```python
from build123d import *

# Parameters (mm, degrees)
BOSS_EXTRUDE1_DEPTH     = 7
BOSS_EXTRUDE2_OUTLINE_R = 32.5
BOSS_EXTRUDE2_DEPTH     = 5
CUT_EXTRUDE1_START      = -10
CUT_EXTRUDE1_DEPTH      = 10
CIRPATTERN1_COUNT       = 12


# Read off the part's stored shape, not the designer's step: Boss-Extrude2, CBORE for M3 SHCS1
with BuildPart() as part:
    # Sketch1 → Boss-Extrude1 (new body)
    with BuildSketch(Plane.XY):
        with BuildLine():
            Line((0, 0), (-0.403978912, 15.69480172))
            ThreePointArc((-0.403978912, 15.69480172), (-9.850874058, 16.938509061), (-18.653978912, 20.584874482))
            ThreePointArc((-18.653978912, 20.584874482), (-20.11149054, 20.82324131), (-21.567676923, 20.576907974))
            ThreePointArc((-21.567676923, 20.576907974), (-24.205855638, 20.575365577), (-26.541253498, 21.802519254))
            ThreePointArc((-26.541253498, 21.802519254), (-28.493972378, 23.657335535), (-30.31737883, 25.639416102))
            ThreePointArc((-30.31737883, 25.639416102), (-31.544532507, 27.974813962), (-31.54299011, 30.612992677))
            ThreePointArc((-31.54299011, 30.612992677), (-31.455305934, 32.324569937), (-32.01390615, 33.94480172))
            Line((-32.01390615, 33.94480172), (-51.738215412, 33.94480172))
            ThreePointArc((-51.738215412, 33.94480172), (-38.72021408, 13.062776736), (-17.866169147, 0))
            Line((-17.866169147, 0), (0, 0))
        make_face()
        with BuildLine():
            ThreePointArc((17.846021088, 20.584874482), (9.042916235, 16.938509061), (-0.403978912, 15.69480172))
            Line((-0.403978912, 15.69480172), (0, 0))
            Line((0, 0), (17.866169147, 0))
            ThreePointArc((17.866169147, 0), (38.72021408, 13.062776736), (51.738215412, 33.94480172))
            Line((51.738215412, 33.94480172), (31.205948327, 33.94480172))
            ThreePointArc((31.205948327, 33.94480172), (30.756396425, 32.859487423), (30.603062644, 31.69480172))
            ThreePointArc((30.603062644, 31.69480172), (30.636176894, 31.149887325), (30.735032287, 30.612992677))
            ThreePointArc((30.735032287, 30.612992677), (30.855855546, 29.956788108), (30.896328518, 29.290781625))
            ThreePointArc((30.896328518, 29.290781625), (30.537924024, 27.337836245), (29.509421007, 25.639416102))
            ThreePointArc((29.509421007, 25.639416102), (27.880292336, 23.910530473), (26.151406706, 22.281401802))
            ThreePointArc((26.151406706, 22.281401802), (23.816008846, 21.054248125), (21.177830131, 21.055790522))
            ThreePointArc((21.177830131, 21.055790522), (19.466252872, 21.143474697), (17.846021088, 20.584874482))
        make_face()
    extrude(amount=BOSS_EXTRUDE1_DEPTH)

    # Boss-Extrude2 outline → Boss-Extrude2 (add)
    with BuildSketch(Plane.XY.offset(7)):
        with BuildLine():
            Line((-17.866169147, 0), (17.866169147, 0))
            ThreePointArc((17.866169147, 0), (0, 106.4), (-17.866169147, 0))
        make_face()
        with Locations((0, 51.7)):
            Circle(BOSS_EXTRUDE2_OUTLINE_R, mode=Mode.SUBTRACT)
    extrude(amount=BOSS_EXTRUDE2_DEPTH)

    # Sketch4 → Cut-Extrude1 (cut)
    with BuildSketch(Plane.XY.offset(12).offset(CUT_EXTRUDE1_START)):
        with BuildLine():
            ThreePointArc((51.738215412, 33.94480172), (-1.913911899, 106.366506576), (-50.369813341, 30.369929583))
            Line((-50.369813341, 30.369929583), (-49.282026095, 30.369929583))
            ThreePointArc((-49.282026095, 30.369929583), (-1.919212398, 105.365693173), (50.679807952, 33.94480172))
            Line((50.679807952, 33.94480172), (51.738215412, 33.94480172))
        make_face()
    extrude(amount=CUT_EXTRUDE1_DEPTH, mode=Mode.SUBTRACT)

    # CBORE for M3 SHCS1 outline → CBORE for M3 SHCS1 (revolve, cut)
    with BuildSketch(Plane(origin=(10, 5, 0), x_dir=(1, 0, 0), z_dir=(0, -1, 0))):
        Polygon((0, 0), (1.6, 0), (1.6, 9), (3.25, 9), (3.25, 11.975), (3.275, 12), (0, 12), align=None)
    revolve(axis=Axis((10, 5, 0), (0, 0, 1)), mode=Mode.SUBTRACT)

    # CBORE for M3 SHCS1 2 outline → CBORE for M3 SHCS1 2 (revolve, cut)
    with BuildSketch(Plane(origin=(-10, 5, 0), x_dir=(1, 0, 0), z_dir=(0, -1, 0))):
        Polygon((0, 12), (0, 0), (1.6, 0), (1.6, 9), (3.25, 9), (3.25, 11.975), (3.275, 12), align=None)
    revolve(axis=Axis((-10, 5, 0), (0, 0, 1)), mode=Mode.SUBTRACT)

    # Sketch10 → CBORE for M4 SHCS2 (revolve, cut)
    with BuildSketch(Plane(origin=(0, 97.4, 12), x_dir=(0, -1, 0), z_dir=(1, 0, 0))):
        Polygon((0, 0), (0, 12), (2.25, 12), (2.25, 4), (4, 4), (4, 0.025), (4.025, 0), align=None)
    cbore_for_m4_shcs2 = revolve(axis=Axis((0, 97.4, 18.35), (0, 0, -1)), mode=Mode.SUBTRACT)

    # CirPattern1: CBORE for M4 SHCS2 ×12 about axis
    cirpattern1_axis = Axis((0, 51.7, 0), (0, 0, 1))
    for i in range(1, CIRPATTERN1_COUNT):
        add(cbore_for_m4_shcs2.rotate(cirpattern1_axis, i * 360 / CIRPATTERN1_COUNT), mode=Mode.SUBTRACT)


solid = part.part
```
Geometry: final body of the model. Coordinates: model frame, mm. A direction names the side the tool comes from. Give positions to 0.01 mm unless a question says otherwise; leave off trailing zeros. Order: outer loops, then holes, each group sorted by start corner. A loop starts at its lowest first (then second) coordinate and runs counter-clockwise, first axis right, second up. Notation, with made-up numbers: (63.5, -5) -> (73.5, -5) arc R7 cw to (73.5, -1) -> close; hole circle Ø2 at (13, -24). An arc over 180 degrees is marked (long way). Write each question's results on one line, items separated by ' | '. Start each with the question number.
1) Section C-C (z = 10.5). Count the separate pieces of the cut face and the enclosed holes in it, then the cut area to 3 significant figures.
2) Draft query along Y for faces 1 (the flat face through (-1, 13, 0)), 2 (the cylindrical face through (-42.95, 26.7, 10.02)), 3 (the cylindrical face through (-28.468, 23.63, 3.451)). Return one class per face: pulls with the +Y half, pulls with the -Y half, needs draft (parallel to the pull), parting line crosses it, or undercut.
3) Section B-B (x = 10). Return loops of the section in (y, z) (3 decimals).
4) Section A-A (x = 45.7). Return loops of the section in (y, z) (3 decimals).
5) Set-up query: faces 4 (the cylindrical face through (-31.535, 27.939, 3.451)), 5 (the flat face through (8.6, 3.6, 9)), 6 (the cylindrical face through (-24.17, 20.567, 3.451)). Return all of +Z, -Z, +X, -X, +Y, -Y with unobstructed straight access to the full face (end or side cutting, diameter ignored); none if empty.
6) Line query: line 1 (X direction, y = 90, z = 11); line 2 (X direction, y = 74.55, z = 7.4); line 3 (Y direction, x = -22.85, z = 8.85). Output: solid intervals per line, ascending. Write a range as from..to.
7) First-contact query: pin 1 (4 mm diameter, centred on x = 44.5, y = 50, fed in from +Z); pin 2 (4 mm diameter, centred on x = -41, y = 74.5, fed in from +Z); pin 3 (10.5 mm diameter, centred on x = -39.58, y = 74.55, fed in from -Z); pin 4 (2 mm diameter, centred on y = 24, z = 2.5, fed in from -X). Flat tips, straight axial feed; report the tip coordinate or a pass-through.
Calculated:
1) separate pieces: 1 | enclosed holes: 15 | area: 5,130 mm2
2) face 1: needs draft | face 2: undercut | face 3: pulls with the +Y half
3) outline: (0, 0) -> (3.4, 0) -> (3.4, 9) -> (1.75, 9) -> (1.75, 11.975) -> (1.725, 12) -> (0, 12) -> close; (6.6, 0) -> (17.209, 0) -> (17.209, 7) -> (20.777, 7) -> (20.777, 12) -> (8.275, 12) -> (8.25, 11.975) -> (8.25, 9) -> (6.6, 9) -> close; (82.623, 7) -> (104.461, 7) -> (104.461, 12) -> (82.623, 12) -> close
4) outline: (21.64, 0) -> (33.945, 0) -> (33.945, 7) -> (49.45, 7) -> (49.45, 8) -> (47.7, 8) -> (47.7, 11.975) -> (47.675, 12) -> (21.64, 12) -> close; (53.95, 7) -> (79.899, 7) -> (79.899, 12) -> (55.725, 12) -> (55.7, 11.975) -> (55.7, 8) -> (53.95, 8) -> close
5) face 4: -Z | face 5: +Z | face 6: -Z, +Y
6) line 1: -37.64..-26.64, -19.06..19.06, 26.64..37.64 | line 2: -48.6..-41.83, -37.33..-23.11, 23.11..37.33, 41.83..48.6 | line 3: 2..8.12, 16.12..28.59, 74.81..87.28, 95.28..100.3
7) pin 1: z = 12 | pin 2: z = 8 | pin 3: z = 7 | pin 4: x = -47.74
